from build123d import *

# Parameters (mm, degrees)
SKETCH_1_W               = 65
SKETCH_1_H               = 60
EXTRUDE_1_DEPTH          = 2
SKETCH_2_R               = 1.5
CUT_EXTRUDE_1_DEPTH      = 2
SKETCH_3_R               = 1.5
CUT_EXTRUDE_2_DEPTH      = 45.274710615
MIRROR_2_COPY_1_SKETCH_R = 1.5
MIRROR_2_COPY_1_DEPTH    = 2
MIRROR_2_COPY_2_SKETCH_R = 1.5
MIRROR_2_COPY_2_DEPTH    = 45.274710615
SKETCH_4_W               = 10
SKETCH_4_H               = 34
CUT_EXTRUDE_3_DEPTH      = 45.274710615
MIRROR_4_COPY_1_SKETCH_W = 10
MIRROR_4_COPY_1_SKETCH_H = 34
MIRROR_4_COPY_1_DEPTH    = 45.274710615
SKETCH_5_R               = 7
CUT_EXTRUDE_4_DEPTH      = 45.274710615
FILLET_1_R               = 3
MIRROR_6_DEPTH           = 2
SKETCH_6_R               = 1.5
CUT_EXTRUDE_5_DEPTH      = 45.274710615
CUT_EXTRUDE_6_DEPTH      = 45.274710615
MIRROR_8_COPY_1_SKETCH_R = 1.5
MIRROR_8_COPY_1_DEPTH    = 45.274710615
FILLET_2_R               = 3


# Read off the part's stored shape, not the designer's step: 镜向6
with BuildPart() as part:
    # 草图1 → 凸台-拉伸1 (new body)
    with BuildSketch(Plane(origin=(0, 0, 0), x_dir=(1, 0, 0), z_dir=(0, 1, 0))):
        Rectangle(SKETCH_1_W, SKETCH_1_H)
    extrude(amount=EXTRUDE_1_DEPTH)

    # 草图2 → 切除-拉伸1 (cut)
    with BuildSketch(Plane(origin=(0, 2, 0), x_dir=(1, 0, 0), z_dir=(0, 1, 0))):
        with Locations(Location((-28.367832783, 25, 0), (0, 0, 270))):
            Circle(SKETCH_2_R)
    cut_extrude_1 = extrude(amount=-CUT_EXTRUDE_1_DEPTH, mode=Mode.SUBTRACT)

    # 草图3 → 切除-拉伸2 (cut, through all)
    with BuildSketch(Plane(origin=(0, 2, 0), x_dir=(1, 0, 0), z_dir=(0, 1, 0))):
        with Locations(Location((-5.617832783, 25, 0), (0, 0, 270))):
            Circle(SKETCH_3_R)
    cut_extrude_2 = extrude(amount=-CUT_EXTRUDE_2_DEPTH, mode=Mode.SUBTRACT)

    # 镜向1: 切除-拉伸1, 切除-拉伸2 across plane
    add(cut_extrude_1.mirror(Plane(origin=(0, 0, 0), x_dir=(0, 0, 1), z_dir=(1, 0, 0))), mode=Mode.SUBTRACT)
    add(cut_extrude_2.mirror(Plane(origin=(0, 0, 0), x_dir=(0, 0, 1), z_dir=(1, 0, 0))), mode=Mode.SUBTRACT)

    # 镜向2: 切除-拉伸1, 切除-拉伸2 across plane
    add(cut_extrude_1.mirror(Plane.XY), mode=Mode.SUBTRACT)
    add(cut_extrude_2.mirror(Plane.XY), mode=Mode.SUBTRACT)

    # 镜向2 copy 1 sketch → 镜向2 copy 1 (cut)
    with BuildSketch(Plane(origin=(0, 2, 0), x_dir=(-1, 0, 0), z_dir=(0, 1, 0))):
        with Locations(Location((-28.367832783, 25, 0), (0, 0, 270))):
            Circle(MIRROR_2_COPY_1_SKETCH_R)
    extrude(amount=-MIRROR_2_COPY_1_DEPTH, mode=Mode.SUBTRACT)

    # 镜向2 copy 2 sketch → 镜向2 copy 2 (cut, through all)
    with BuildSketch(Plane(origin=(0, 2, 0), x_dir=(-1, 0, 0), z_dir=(0, 1, 0))):
        with Locations(Location((-5.617832783, 25, 0), (0, 0, 270))):
            Circle(MIRROR_2_COPY_2_SKETCH_R)
    extrude(amount=-MIRROR_2_COPY_2_DEPTH, mode=Mode.SUBTRACT)

    # 草图4 → 切除-拉伸3 (cut, through all)
    with BuildSketch(Plane(origin=(0, 2, 0), x_dir=(1, 0, 0), z_dir=(0, 1, 0))):
        with Locations((-16.992832783, 25)):
            Rectangle(SKETCH_4_W, SKETCH_4_H)
    cut_extrude_3 = extrude(amount=-CUT_EXTRUDE_3_DEPTH, mode=Mode.SUBTRACT)

    # 镜向3: 切除-拉伸3 across plane
    add(cut_extrude_3.mirror(Plane.XY), mode=Mode.SUBTRACT)

    # 镜向4: 切除-拉伸3 across plane
    add(cut_extrude_3.mirror(Plane(origin=(0, 0, 0), x_dir=(0, 0, 1), z_dir=(1, 0, 0))), mode=Mode.SUBTRACT)

    # 镜向4 copy 1 sketch → 镜向4 copy 1 (cut, through all)
    with BuildSketch(Plane(origin=(0, 2, 0), x_dir=(-1, 0, 0), z_dir=(0, 1, 0))):
        with Locations((-16.992832783, 25)):
            Rectangle(MIRROR_4_COPY_1_SKETCH_W, MIRROR_4_COPY_1_SKETCH_H)
    extrude(amount=-MIRROR_4_COPY_1_DEPTH, mode=Mode.SUBTRACT)

    # 草图5 → 切除-拉伸4 (cut, through all)
    with BuildSketch(Plane(origin=(0, 2, 0), x_dir=(1, 0, 0), z_dir=(0, 1, 0))):
        with Locations(Location((0, 0, 0), (0, 0, 270))):
            Circle(SKETCH_5_R)
    extrude(amount=-CUT_EXTRUDE_4_DEPTH, mode=Mode.SUBTRACT)

    # 圆角1
    fillet_1_edges = [part.edges().sort_by_distance(p)[0] for p in [
        (-21.992832783, 1, 30),
        (-11.992832783, 1, 30),
        (32.5, 1, 30),
        (-32.5, 1, 30),
        (21.992832783, 1, 30),
        (11.992832783, 1, 30),
    ]]
    fillet(fillet_1_edges, radius=FILLET_1_R)

    # 镜向6 outline → 镜向6 (cut)
    with BuildSketch(Plane(origin=(0, 0, 0), x_dir=(1, 0, 0), z_dir=(0, 1, 0))):
        with BuildLine():
            Line((-11.992832783, 30), (-11.992832783, 27))
            ThreePointArc((-11.992832783, 27), (-11.114153127, 29.121320343), (-8.992832783, 30))
            Line((-8.992832783, 30), (-11.992832783, 30))
        make_face()
        with BuildLine():
            Line((11.992832783, 30), (8.992832783, 30))
            ThreePointArc((8.992832783, 30), (11.114153127, 29.121320343), (11.992832783, 27))
            Line((11.992832783, 27), (11.992832783, 30))
        make_face()
        with BuildLine():
            Line((32.5, 30), (29.5, 30))
            ThreePointArc((29.5, 30), (31.621320344, 29.121320344), (32.5, 27))
            Line((32.5, 27), (32.5, 30))
        make_face()
        with BuildLine():
            ThreePointArc((21.992832783, 27), (22.871512439, 29.121320344), (24.992832783, 30))
            Line((24.992832783, 30), (21.992832783, 30))
            Line((21.992832783, 30), (21.992832783, 27))
        make_face()
        with BuildLine():
            ThreePointArc((-32.5, 27), (-31.621320344, 29.121320344), (-29.5, 30))
            Line((-29.5, 30), (-32.5, 30))
            Line((-32.5, 30), (-32.5, 27))
        make_face()
        with BuildLine():
            ThreePointArc((-24.992832783, 30), (-22.871512439, 29.121320344), (-21.992832783, 27))
            Line((-21.992832783, 27), (-21.992832783, 30))
            Line((-21.992832783, 30), (-24.992832783, 30))
        make_face()
    extrude(amount=MIRROR_6_DEPTH, mode=Mode.SUBTRACT)

    # 草图6 → 切除-拉伸5 (cut, through all)
    with BuildSketch(Plane(origin=(0, 2, 0), x_dir=(1, 0, 0), z_dir=(0, 1, 0))):
        with Locations(Location((-28.367832783, -9, 0), (0, 0, 270))):
            Circle(SKETCH_6_R)
    cut_extrude_5 = extrude(amount=-CUT_EXTRUDE_5_DEPTH, mode=Mode.SUBTRACT)

    # 镜向7: 切除-拉伸5 across plane
    add(cut_extrude_5.mirror(Plane.XY), mode=Mode.SUBTRACT)

    # 草图7 → 切除-拉伸6 (cut, through all)
    with BuildSketch(Plane(origin=(0, 2, 0), x_dir=(1, 0, 0), z_dir=(0, 1, 0))):
        with BuildLine():
            Line((-11.509285997, 1.5), (-21.509285997, 1.5))
            ThreePointArc((-21.509285997, 1.5), (-23.009285997, 0), (-21.509285997, -1.5))
            Line((-21.509285997, -1.5), (-11.509285997, -1.5))
            ThreePointArc((-11.509285997, -1.5), (-10.009285997, 0), (-11.509285997, 1.5))
        make_face()
    cut_extrude_6 = extrude(amount=-CUT_EXTRUDE_6_DEPTH, mode=Mode.SUBTRACT)

    # 镜向8: 切除-拉伸5, 切除-拉伸6 across plane
    add(cut_extrude_5.mirror(Plane(origin=(0, 0, 0), x_dir=(0, 0, 1), z_dir=(1, 0, 0))), mode=Mode.SUBTRACT)
    add(cut_extrude_6.mirror(Plane(origin=(0, 0, 0), x_dir=(0, 0, 1), z_dir=(1, 0, 0))), mode=Mode.SUBTRACT)

    # 镜向8 copy 1 sketch → 镜向8 copy 1 (cut, through all)
    with BuildSketch(Plane(origin=(0, 2, 0), x_dir=(-1, 0, 0), z_dir=(0, 1, 0))):
        with Locations(Location((-28.367832783, -9, 0), (0, 0, 270))):
            Circle(MIRROR_8_COPY_1_SKETCH_R)
    extrude(amount=-MIRROR_8_COPY_1_DEPTH, mode=Mode.SUBTRACT)

    # 圆角2
    fillet_2_edges = [part.edges().sort_by_distance(p)[0] for p in [
        (11.992832783, 1, -8),
        (21.992832783, 1, -8),
        (-21.992832783, 1, -8),
        (-11.992832783, 1, -8),
        (-11.992832783, 1, 8),
        (-21.992832783, 1, 8),
        (21.992832783, 1, 8),
        (11.992832783, 1, 8),
    ]]
    fillet(fillet_2_edges, radius=FILLET_2_R)


solid = part.part
CAD build for the part. Positions are in the model's coordinates, mm. A direction names the side the tool comes from. Coordinates: 2 decimals unless noted, no trailing zeros. Loops run counter-clockwise (first coordinate to the right, second up) from the corner with the lowest first, then second, coordinate; pieces in that order, holes last. Notation, with made-up numbers: (12, 45.5) -> (56, 45.5) arc R15 cw to (56, 59.5) -> close; hole circle Ø5 at (52, 76.25). An arc over 180 degrees is marked (long way). One line per item, written item: value.
1. Slice it at B-B on z = 0. Write the cut outline in (x, y).
Answers:
outline: (-32.5, 0) -> (-23.01, 0) -> (-23.01, 2) -> (-32.5, 2) -> close; (-10.01, 0) -> (-7, 0) -> (-7, 2) -> (-10.01, 2) -> close; (7, 0) -> (10.01, 0) -> (10.01, 2) -> (7, 2) -> close; (23.01, 0) -> (32.5, 0) -> (32.5, 2) -> (23.01, 2) -> close
2. Slice it at A-A on z = 25. Write the cut outline in (x, y), and give its area (3 significant figures).
Answers:
outline: (-32.5, 0) -> (-29.87, 0) -> (-29.87, 2) -> (-32.5, 2) -> close; (-26.87, 0) -> (-21.99, 0) -> (-21.99, 2) -> (-26.87, 2) -> close; (-11.99, 0) -> (-7.12, 0) -> (-7.12, 2) -> (-11.99, 2) -> close; (-4.12, 0) -> (4.12, 0) -> (4.12, 2) -> (-4.12, 2) -> close; (7.12, 0) -> (11.99, 0) -> (11.99, 2) -> (7.12, 2) -> close; (21.99, 0) -> (26.87, 0) -> (26.87, 2) -> (21.99, 2) -> close; (29.87, 0) -> (32.5, 0) -> (32.5, 2) -> (29.87, 2) -> close
area: 66.0 mm^2
3. Pull direction X, two halves, no side cores. Call faces 4 (the face through (-10.01, 1.01, 0.03)), 5 (the face through (27, 1, -30)), 6 (the face through (31.6, 1.01, 29.14)): pulls with the +X half, pulls with the -X half, needs draft (parallel to the pull), parting line crosses it, or undercut.
Answers:
face 4: undercut
face 5: needs draft
face 6: pulls with the +X half
4. Flat gauge pin, fed straight in: P1, Ø1, axis at x = -17.5, y = 1.5, coming from the -Z side. Where does the tip first touch, or does it go through?
Answers:
P1: stops at z = -8
5. Which spindle directions (+Z, -Z, +X, -X, +Y, -Y) get a long thin tool onto all of the face, cutting with end or side? Do faces 1 (the face through (17, 1, 8)), 2 (the face through (-12.89, 0.99, -8.86)), 3 (the face through (-5.6, 1, 26.5)). Say none if no direction does.
Answers:
face 1: +Z, +Y, -Y
face 2: -Z, +Y, -Y
face 3: +Y, -Y
6. Slice it at D-D on z = 9. Write the cut outline in (x, y), and give its area (3 significant figures).
Answers:
outline: (-32.5, 0) -> (-29.87, 0) -> (-29.87, 2) -> (-32.5, 2) -> close; (-26.87, 0) -> (-21.23, 0) -> (-21.23, 2) -> (-26.87, 2) -> close; (-12.76, 0) -> (12.76, 0) -> (12.76, 2) -> (-12.76, 2) -> close; (21.23, 0) -> (26.87, 0) -> (26.87, 2) -> (21.23, 2) -> close; (29.87, 0) -> (32.5, 0) -> (32.5, 2) -> (29.87, 2) -> close
area: 84.1 mm^2
7. Drill centre lines: line 1 (X direction, y = 1.25, z = 21.5); line 2 (X direction, y = 0.8, z = 9); line 3 (Z direction, x = 4.5, y = 0.8). Where is each one in solid material? Low to high. Write a range as [from, to].
Answers:
line 1: x = [-32.5, -21.99], [-11.99, 11.99], [21.99, 32.5]
line 2: x = [-32.5, -29.87], [-26.87, -21.23], [-12.76, 12.76], [21.23, 26.87], [29.87, 32.5]
line 3: z = [-30, -26], [-24, -5.36], [5.36, 24], [26, 30]
8. Slice it at C-C on x = -13.5. Write the cut outline in (y, z), and give its area (3 significant figures).
Answers:
outline: (0, -8.4) -> (2, -8.4) -> (2, -1.5) -> (0, -1.5) -> close; (0, 1.5) -> (2, 1.5) -> (2, 8.4) -> (0, 8.4) -> close
area: 27.6 mm^2
